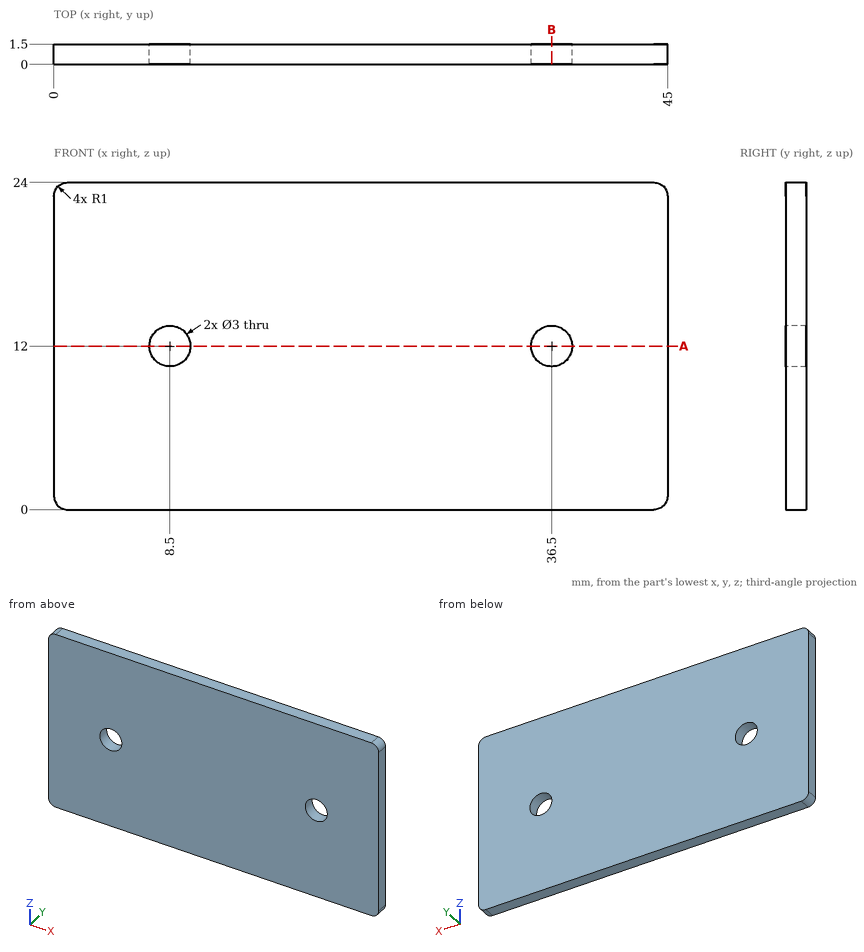
Here's the drawing with two shaded views (mm, measured from the low corner). I have some questions. Coordinates: 2 decimals unless noted, no trailing zeros. Order: outer loops, then holes, each group sorted by start corner. A loop starts at its lowest first (then second) coordinate and runs counter-clockwise, first axis right, second up. Notation, with made-up numbers: M 0.25,59.5 L 55.25,59.5 A27 cw 55.25,93.5 Z; hole C 7,0 d1. An arc over 180 degrees is marked long. Answer as CSV lines item,"result".
Item 1: Imagine slicing it at B-B on x = 36.5. Write out the boundary of the cut face in (y, z), plus the area to 3 significant figures.
Results found:
outline,"M 0,0 L 1.5,0 L 1.5,10.5 L 0,10.5 Z; M 0,13.5 L 1.5,13.5 L 1.5,24 L 0,24 Z"
area,"31.5 mm2"
Item 2: For pin 1 (1.8 mm diameter, centred on x = 36.5, z = 12, fed in from -Y); pin 2 (8 mm diameter, centred on x = 34, z = 15.5, fed in from -Y), each with a flat end and sliding along its axis, tell me the tip position at first contact or that it passes through.
Results found:
pin 1,"through"
pin 2,"y = 0"
Item 3: Imagine slicing it at A-A on z = 12. Write out the boundary of the cut face in (x, y), plus the area to 3 significant figures.
Results found:
outline,"M 0,0 L 7,0 L 7,1.5 L 0,1.5 Z; M 10,0 L 35,0 L 35,1.5 L 10,1.5 Z; M 38,0 L 45,0 L 45,1.5 L 38,1.5 Z"
area,"58.5 mm2"
Item 4: If I drill on line 1 (X direction, y = 0.7, z = 12); line 2 (Z direction, x = 36.5, y = 1.2), over which ranges is the centre line in solid material (lowest first)?
Results found:
line 1,"0 to 7, 10 to 35, 38 to 45"
line 2,"0 to 10.5, 13.5 to 24"
